```python
from build123d import *

# Parameters (mm, degrees)
SKETCH1_W          = 50
SKETCH1_H          = 200
SKETCH2_R          = 45
CUT_EXTRUDE1_DEPTH = 195
FILLET2_R          = 2
FILLET3_R          = 2


with BuildPart() as part:
    # Sketch1 → Revolve1 (revolve)
    with BuildSketch(Plane.XY, mode=Mode.PRIVATE) as revolve1_sk:
        with Locations((-25, -134.703470817)):
            Rectangle(SKETCH1_W, SKETCH1_H)
    revolve(revolve1_sk.sketch.rotate(Axis((0, 0, 0), (0, -1, 0)), 270), axis=Axis((0, 0, 0), (0, -1, 0)))

    # Sketch2 → Cut-Extrude1 (cut)
    with BuildSketch(Plane(origin=(0, -34.703470817, 0), x_dir=(1, 0, 0), z_dir=(0, 1, 0))):
        with Locations(Location((0, 0, 0), (0, 0, 270))):
            Circle(SKETCH2_R)
    extrude(amount=-CUT_EXTRUDE1_DEPTH, mode=Mode.SUBTRACT)

    # Fillet2
    fillet2_edges = [part.edges().sort_by_distance(p)[0] for p in [
        (0, -34.703470817, -50),
        (0, -34.703470817, -45),
    ]]
    fillet(fillet2_edges, radius=FILLET2_R)

    # Fillet3
    fillet3_edges = [part.edges().sort_by_distance(p)[0] for p in [
        (0, -234.703470817, -50),
    ]]
    fillet(fillet3_edges, radius=FILLET3_R)


solid = part.part
```
Input: part model. Units: mm. Frame: model coordinates. Give positions to 0.01 mm unless a question says otherwise; leave off trailing zeros. Order: outer loops, then holes, each group sorted by start corner. A loop starts at its lowest first (then second) coordinate and runs counter-clockwise, first axis right, second up. Notation, with made-up numbers: (-7, 72) - (47, 72) arc R20 ccw to (47, 83) - close; hole circle Ø2 at (-16, -22.5). An arc over 180 degrees is marked (long way). Put each result on its own line as item: value.
Item 1: Ray query, L1, parallel to X at y = -81, z = 0; L2, parallel to Y at x = 41, z = -1; L3, parallel to X at y = -153, z = -36. Return the intervals inside material, ascending. Write a range as from..to.
Found:
L1: x = -50..-45, 45..50
L2: y = -234.7..-229.7
L3: x = -34.7..-27, 27..34.7
Item 2: Draft query along X for faces 1 (the flat face through (1, -229.703, -1)), 2 (the flat face through (-1, -234.703, -1)), 3 (the cylindrical face through (-17.235, -131.852, 41.569)), 4 (the cylindrical face through (-15.02, -133.33, 47.69)). Return one class per face: +X half, -X half, draft (parallel to the pull), parting line (faces both ways), or undercut.
Found:
face 1: undercut
face 2: draft
face 3: undercut
face 4: parting line
Item 3: Section query C-C, the plane y = -72.5. Return loops of the section in (x, z), then the cut area to 3 significant figures.
Found:
outline: circle Ø100 at (0, 0); hole circle Ø90 at (0, 0)
area: 1,490 mm^2
Item 4: Section query B-B, the plane x = 0. Return loops of the section in (y, z).
Found:
outline: (-234.7, -48) arc R2 ccw to (-232.7, -50) - (-36.7, -50) arc R2 ccw to (-34.7, -48) - (-34.7, -47) arc R2 ccw to (-36.7, -45) - (-229.7, -45) - (-229.7, 45) - (-36.7, 45) arc R2 ccw to (-34.7, 47) - (-34.7, 48) arc R2 ccw to (-36.7, 50) - (-232.7, 50) arc R2 ccw to (-234.7, 48) - close
Item 5: Contact query for flat-ended pins moving along their axis: pin 1 (4 mm diameter, centred on x = -28.5, z = -5.5, fed in from +Y); pin 2 (5 mm diameter, centred on y = -88.5, z = 0.5, fed in from +X); pin 3 (12 mm diameter, centred on x = 33, y = -92.5, fed in from -Z). Output: stop coordinate, or through.
Found:
pin 1: stops at y = -229.7
pin 2: stops at x = 50
pin 3: stops at z = -42.08
Item 6: Section query A-A, the plane z = 0. Return loops of the section in (x, y).
Found:
outline: (-50, -232.7) arc R2 ccw to (-48, -234.7) - (48, -234.7) arc R2 ccw to (50, -232.7) - (50, -36.7) arc R2 ccw to (48, -34.7) - (47, -34.7) arc R2 ccw to (45, -36.7) - (45, -229.7) - (-45, -229.7) - (-45, -36.7) arc R2 ccw to (-47, -34.7) - (-48, -34.7) arc R2 ccw to (-50, -36.7) - close
